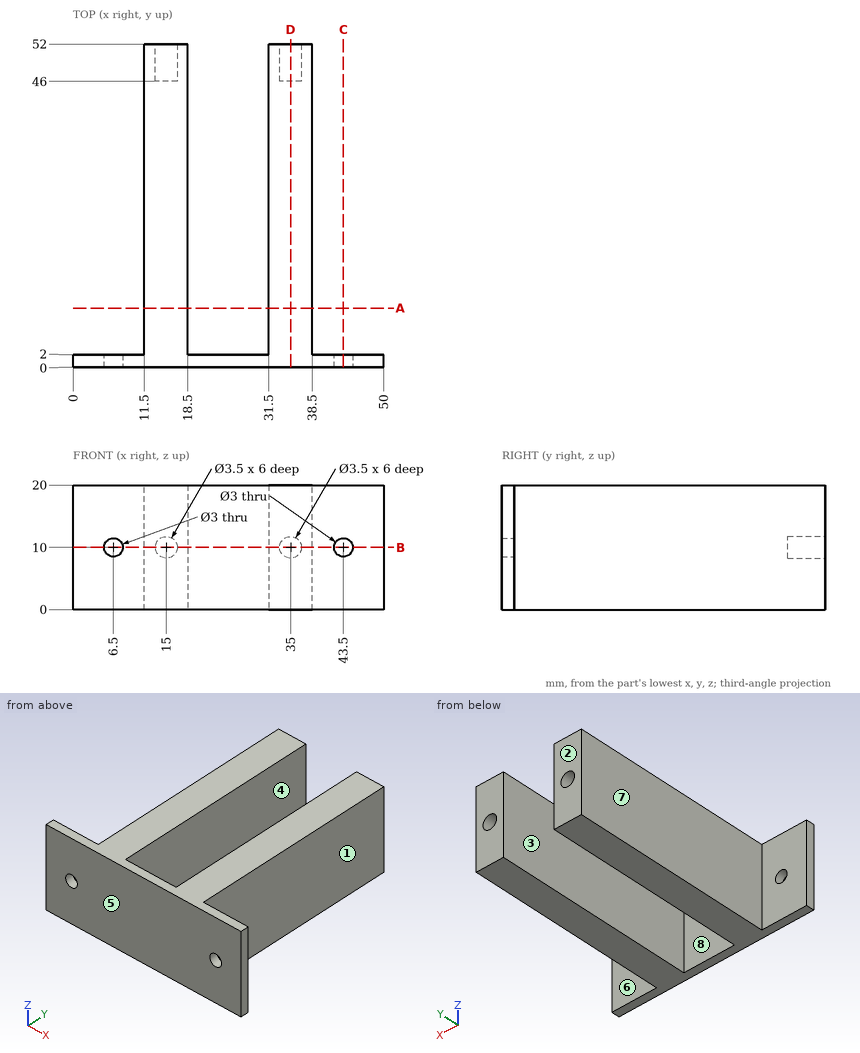
Can you work these out from the drawing? Everything is in mm from the part's minimum corner. A direction names the side the tool comes from. Coordinates: 2 decimals unless noted, no trailing zeros. Loops run counter-clockwise (first coordinate to the right, second up) from the corner with the lowest first, then second, coordinate; pieces in that order, holes last.
1) Imagine slicing it at B-B on z = 10. List the corners of the cut face in (x, y) for me.
2) Imagine slicing it at C-C on x = 43.5. List the corners of the cut face in (y, z) for me, plus the area to 3 significant figures.
3) Which directions (+Z, -Z, +X, -X, +Y, -Y) give clear straight access to the entire face, cutting with the end or side of a thin tool? Please do the marked faces 5, 6, 7 and 8.
4) Imagine slicing it at A-A on y = 9.5. List the corners of the cut face in (x, z) for me, plus the area to 3 significant figures.
5) For pin 1 (2.5 mm diameter, centred on x = 43.5, z = 10, fed in from -Y); pin 2 (3 mm diameter, centred on y = 38.5, z = 16.5, fed in from +X); pin 3 (1.8 mm diameter, centred on x = 35.5, z = 10.5, fed in from +Y); pin 4 (6 mm diameter, centred on y = 32, z = 8.5, fed in from -X), each with a flat end and sliding along its axis, tell me the tip position at first contact or that it passes through.
6) I need wall thicknesses on probe 1 along X at (y, z) = (48.6, 10); probe 2 along X at (y, z) = (0.9, 10); probe 3 along X at (y, z) = (17, 1.5). Which ranges of each line are inside material? Lowest first, please.
7) Imagine slicing it at D-D on x = 35. List the corners of the cut face in (y, z) for me, plus the area to 3 significant figures.
8) Thinking about a two-plate mould opening in X: for the marked faces 1, 2, 3 and 4, which applies, pulls with the +X half, pulls with the -X half, needs draft (parallel to the pull), parting line crosses it, or undercut?
Completed:
1. outline: (0, 0) - (5, 0) - (5, 2) - (0, 2) - close; (8, 0) - (42, 0) - (42, 2) - (38.5, 2) - (38.5, 52) - (36.75, 52) - (36.75, 46) - (33.25, 46) - (33.25, 52) - (31.5, 52) - (31.5, 2) - (18.5, 2) - (18.5, 52) - (16.75, 52) - (16.75, 46) - (13.25, 46) - (13.25, 52) - (11.5, 52) - (11.5, 2) - (8, 2) - close; (45, 0) - (50, 0) - (50, 2) - (45, 2) - close
2. outline: (0, 0) - (2, 0) - (2, 8.5) - (0, 8.5) - close; (0, 11.5) - (2, 11.5) - (2, 20) - (0, 20) - close
2. area: 34.0 mm2
3. face 5: +Z, -Z, +X, -X, -Y
3. face 6: +Z, -Z, +X, +Y
3. face 7: +Z, -Z, -X, +Y
3. face 8: +Z, -Z, +Y
4. outline: (11.5, 0) - (18.5, 0) - (18.5, 20) - (11.5, 20) - close; (31.5, 0) - (38.5, 0) - (38.5, 20) - (31.5, 20) - close
4. area: 280 mm2
5. pin 1: passes through
5. pin 2: stops at x = 38.5
5. pin 3: stops at y = 46
5. pin 4: stops at x = 11.5
6. probe 1: x = 11.5 to 13.25, 16.75 to 18.5, 31.5 to 33.25, 36.75 to 38.5
6. probe 2: x = 0 to 5, 8 to 42, 45 to 50
6. probe 3: x = 11.5 to 18.5, 31.5 to 38.5
7. outline: (0, 0) - (52, 0) - (52, 8.25) - (46, 8.25) - (46, 11.75) - (52, 11.75) - (52, 20) - (0, 20) - close
7. area: 1,020 mm2
8. face 1: pulls with the +X half
8. face 2: needs draft
8. face 3: undercut
8. face 4: undercut
